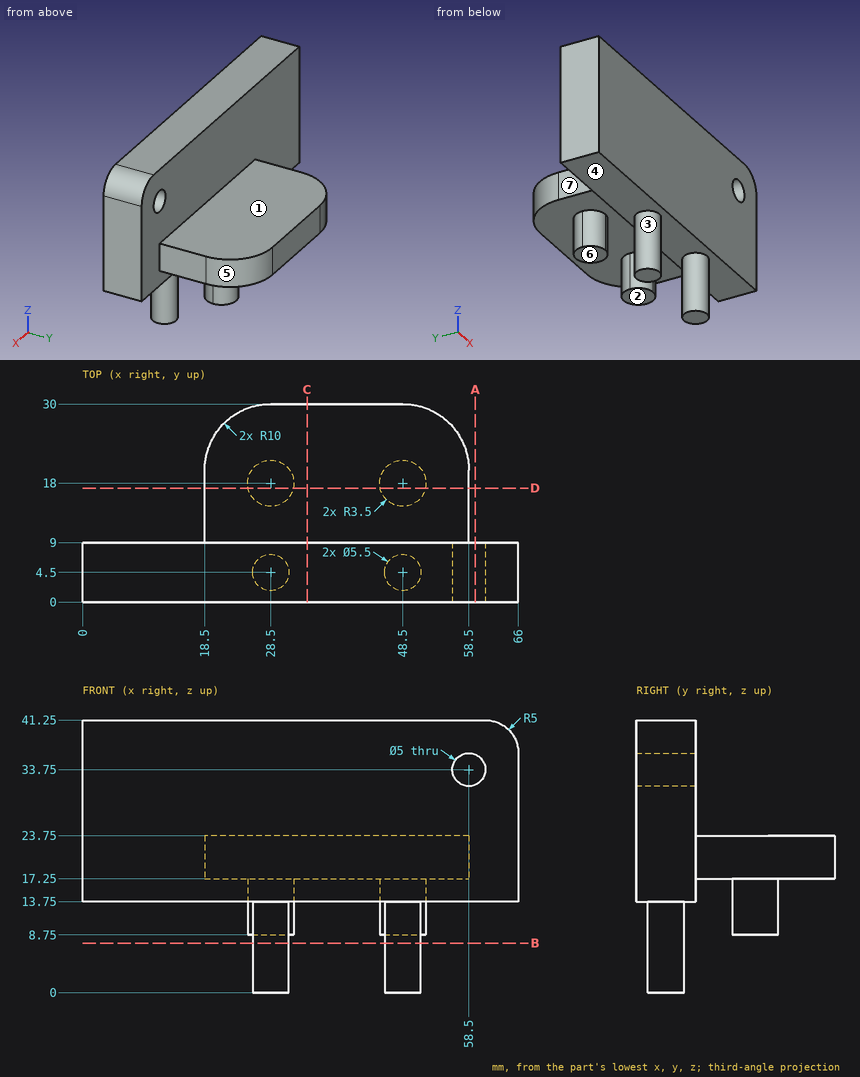
Here's the drawing with two shaded views (mm, measured from the low corner). I have some questions. A direction names the side the tool comes from. Coordinates: 2 decimals unless noted, no trailing zeros. Loops run counter-clockwise (first coordinate to the right, second up) from the corner with the lowest first, then second, coordinate; pieces in that order, holes last. Notation, with made-up numbers: (64.5, 53.25) -> (92.5, 53.25) arc R26 cw to (92.5, 79.25) -> close; hole circle Ø4 at (69.5, 17). An arc over 180 degrees is marked (long way). Answer as a JSON object with one key per item and string values.
1) If I drill on line 1 (X direction, y = 4.75, z = 33.75); line 2 (Z direction, x = 44.5, y = 11.75); line 3 (Y direction, x = 7.5, z = 29), over which ranges is the centre line in solid material (lowest first)?
Results:
{"line 1": "x = 0 to 56, 61 to 66", "line 2": "z = 17.25 to 23.75", "line 3": "y = 0 to 9"}
2) Imagine slicing it at B-B (z = 7.5). Please give me the cut outline in (x, y).
Results:
{"outline": "circle Ø5.5 at (28.5, 4.5); circle Ø5.5 at (48.5, 4.5)"}
3) Imagine slicing it at A-A (x = 59.5). Please give me the cut outline in (y, z).
Results:
{"outline": "(0, 13.75) -> (9, 13.75) -> (9, 31.46) -> (0, 31.46) -> close; (0, 36.04) -> (9, 36.04) -> (9, 41.25) -> (0, 41.25) -> close"}
4) Thinking about a two-plate mould opening in X: for the marked faces 4, 5, 6 and 7, which applies, pulls with the +X half, pulls with the -X half, needs draft (parallel to the pull), parting line crosses it, or undercut?
Results:
{"face 4": "undercut", "face 5": "pulls with the +X half", "face 6": "needs draft", "face 7": "pulls with the -X half"}
5) Imagine slicing it at D-D (y = 17.25). Please give me the cut outline in (x, z), then the cut area to 3 significant figures.
Results:
{"outline": "(18.5, 17.25) -> (25.08, 17.25) -> (25.08, 8.75) -> (31.92, 8.75) -> (31.92, 17.25) -> (45.08, 17.25) -> (45.08, 8.75) -> (51.92, 8.75) -> (51.92, 17.25) -> (58.5, 17.25) -> (58.5, 23.75) -> (18.5, 23.75) -> close", "area": "376 mm^2"}
6) For P1, Ø1, axis at x = 11, y = 8.5, coming from the -Z side; P2, Ø12, axis at x = 32, y = 26, coming from the -Z side; P3, Ø2, axis at y = 17, z = 19, coming from the -X side; P4, Ø8, axis at x = 58, z = 9.5, coming from the -Y side, each with a flat end and sliding along its axis, tell me the tip position at first contact or that it passes through.
Results:
{"P1": "stops at z = 13.75", "P2": "stops at z = 8.75", "P3": "stops at x = 18.5", "P4": "passes through"}
7) Imagine slicing it at C-C (x = 34). Please give me the cut outline in (y, z), then the cut area to 3 significant figures.
Results:
{"outline": "(0, 13.75) -> (9, 13.75) -> (9, 17.25) -> (30, 17.25) -> (30, 23.75) -> (9, 23.75) -> (9, 41.25) -> (0, 41.25) -> close", "area": "384 mm^2"}
8) For the marked faces 1, 2 and 3, which set-ups out of +Z, -Z, +X, -X, +Y, -Y let a thin tool reach every point of the face, with its end or its side?
Results:
{"face 1": "+Z, +X, -X, +Y", "face 2": "-Z, +X, -X, +Y", "face 3": "-Z"}
